Read the model definition and answer for the solid it produces. Units are mm, in the model's axes. Face numbers are marked on the shaded views. A direction names the side the tool comes from. Coordinates: 2 decimals unless noted, no trailing zeros. Write each loop counter-clockwise with the first axis right and the second up, starting at its lowest first coordinate (ties: lowest second). Pieces come first, ordered by that corner, then holes. Notation, with made-up numbers: (16.25, 28) -> (74.25, 28) arc R12 ccw to (74.25, 50) -> close; hole circle Ø1 at (19, -19.5). An arc over 180 degrees is marked (long way). One line per item, written item: value. Start each with the question number.
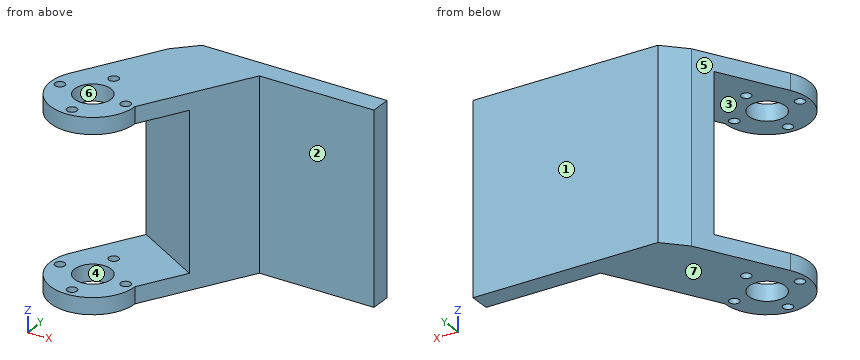
from build123d import *

# Parameters (mm, degrees)
SKETCH1_R           = 4.4
SKETCH1_R_2         = 1.2
BOSS_EXTRUDE1_DEPTH = 46
SKETCH3_W           = 38
SKETCH3_H           = 28
CUT_EXTRUDE2_DEPTH  = 81.708866675
CHAMFER1_SIZE       = 5


with BuildPart() as part:
    # Sketch1 → Boss-Extrude1 (new body)
    with BuildSketch(Plane.XY):
        with BuildLine():
            Line((2.598076211, 25), (-8.876760389, 5.125))
            ThreePointArc((-8.876760389, 5.125), (-2.652895212, -9.900739719), (10.25, 0))
            Line((10.25, 0), (24.68375673, 25))
            Line((24.68375673, 25), (52.598076211, 25))
            Line((52.598076211, 25), (52.598076211, 30))
            Line((52.598076211, 30), (2.598076211, 30))
            Line((2.598076211, 30), (2.598076211, 25))
        make_face()
        Circle(SKETCH1_R, mode=Mode.SUBTRACT)
        with Locations((-8, 0)):
            Circle(SKETCH1_R_2, mode=Mode.SUBTRACT)
        with Locations((0, -8)):
            Circle(SKETCH1_R_2, mode=Mode.SUBTRACT)
        with Locations((8, 0)):
            Circle(SKETCH1_R_2, mode=Mode.SUBTRACT)
        with Locations((0, 8)):
            Circle(SKETCH1_R_2, mode=Mode.SUBTRACT)
    extrude(amount=-BOSS_EXTRUDE1_DEPTH)

    # Sketch3 → Cut-Extrude2 (cut, through all)
    with BuildSketch(Plane(origin=(-8.876760389, 5.125, 0), x_dir=(0, 0, 1), z_dir=(-0.8660254037844363, 0.500000000000004, 0))):
        with Locations((-23, 3.75)):
            Rectangle(SKETCH3_W, SKETCH3_H)
    extrude(amount=-CUT_EXTRUDE2_DEPTH, mode=Mode.SUBTRACT)

    # Chamfer1
    chamfer1_edges = [part.edges().sort_by_distance(p)[0] for p in [
        (2.598076211, 30, -23),
    ]]
    chamfer(chamfer1_edges, length=CHAMFER1_SIZE - 0.0001)  # a hair under: the kernel refuses the full size


solid = part.part
1. A cutting plane is placed at D-D on y = 8. Give the vertices of the cut face in (x, z), then the cut area to 3 significant figures.
2. Given pin 1 (22.5 mm diameter, centred on x = 33.5, z = -22.5, fed in from -Y); pin 2 (12 mm diameter, centred on x = 45.5, y = 14.5, fed in from +Z); pin 3 (6 mm diameter, centred on y = 11, z = -40, fed in from -X); pin 4 (10 mm diameter, centred on y = 10, z = -7, fed in from +X), each flat-ended and moving along its own axis, determine where each tip first touches the part or whether it passes through.
3. Find the intervals of material crossed by probe 1 along Y at (x, z) = (0, -2); probe 2 along Z at (x, y) = (5, -2.5); probe 3 along Y at (x, z) = (8, -43.05), in increasing order. Write a range as from..to.
4. For a pull along X with two mould halves and no side action, classify the marked faces 4, 5, 6 and 7 as +X half, -X half, draft (parallel to the pull), parting line (faces both ways), or undercut.
5. A cutting plane is placed at B-B on y = -2.5. Give the vertices of the cut face in (x, z).
6. A cutting plane is placed at C-C on x = 12. Give the vertices of the cut face in (y, z).
7. A tool of negligible diameter and unlimited length cuts with its end or side. For the marked faces 1, 2 and 3, from which of +Z, -Z, +X, -X, +Y, -Y can it reach the whole face along a straight path? Write none if from no direction.
Derived:
1. outline: (-7.22, -46) -> (-1.2, -46) -> (-1.2, -42) -> (-7.22, -42) -> close; (-7.22, -4) -> (-1.2, -4) -> (-1.2, 0) -> (-7.22, 0) -> close; (1.2, -46) -> (14.87, -46) -> (14.87, -42) -> (1.2, -42) -> close; (1.2, -4) -> (14.87, -4) -> (14.87, 0) -> (1.2, 0) -> close
1. area: 157 mm2
2. pin 1: stops at y = 20.78
2. pin 2: passes through
2. pin 3: stops at x = -6.78
2. pin 4: stops at x = 18.91
3. probe 1: y = -10.25..-9.2, -6.8..-4.4, 4.4..6.8, 9.2..20.5
3. probe 2: z = -46..-42, -4..0
3. probe 3: y = -6.41..-1.2, 1.2..30
4. face 4: undercut
4. face 5: -X half
4. face 6: undercut
4. face 7: draft
5. outline: (-9.94, -46) -> (-3.62, -46) -> (-3.62, -42) -> (-9.94, -42) -> close; (-9.94, -4) -> (-3.62, -4) -> (-3.62, 0) -> (-9.94, 0) -> close; (3.62, -46) -> (9.94, -46) -> (9.94, -42) -> (3.62, -42) -> close; (3.62, -4) -> (9.94, -4) -> (9.94, 0) -> (3.62, 0) -> close
6. outline: (3.03, -46) -> (30, -46) -> (30, 0) -> (3.03, 0) -> (3.03, -4) -> (13.57, -4) -> (13.57, -42) -> (3.03, -42) -> close
7. face 1: +Z, -Z, +X, -X, +Y
7. face 2: +Z, -Z, +X, -Y
7. face 3: -X, -Y
